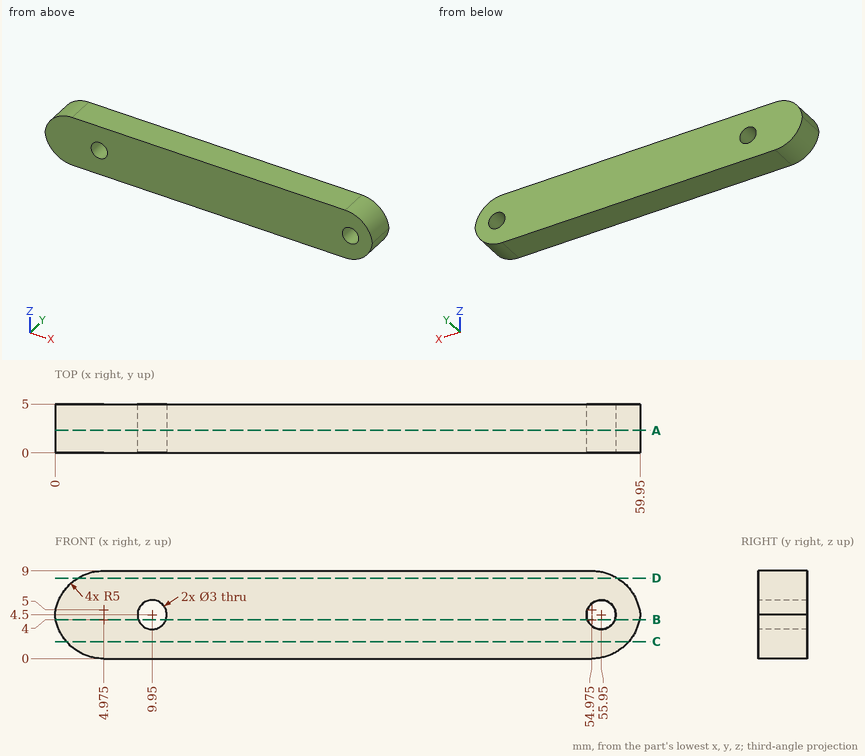
Check sheet for the drawn part. Datum: minimum x, y, z corner. Units: mm. Give positions to 0.01 mm unless a question says otherwise; leave off trailing zeros. Write each loop counter-clockwise with the first axis right and the second up, starting at its lowest first coordinate (ties: lowest second). Pieces come first, ordered by that corner, then holes. Notation, with made-up numbers: M 71,35.5 L 106,35.5 A38 cw 106,74.5 Z; hole C 16.5,-24 d10. An arc over 180 degrees is marked long. One line per question, with ' | ' between items.
1) Gauge pin test, flat ends, axial feed: pin 1 Ø1.5 at (y, z) = (2.5, 7.5) entering from -X; pin 2 Ø5 at (x, z) = (34.5, 5) entering from -Y; pin 3 Ø1.5 at (y, z) = (4.5, 2) entering from -X. Record the tip position at first contact, or that the pin passes through.
Result:
pin 1: stops at x = 0.8 | pin 2: stops at y = 0 | pin 3: stops at x = 0.51
2) Section check C-C on z = 1.75. Enter the section's corners in (x, y), plus the area to 3 significant figures.
Result:
outline: M 1.18,0 L 58.77,0 L 58.77,5 L 1.18,5 Z | area: 288 mm2
3) Section check D-D on z = 8.25. Enter the section's corners in (x, y), plus the area to 3 significant figures.
Result:
outline: M 2.34,0 L 57.61,0 L 57.61,5 L 2.34,5 Z | area: 276 mm2
4) Section check A-A on y = 2.3. Enter the section's corners in (x, z) (3 decimals), plus the area to 3 significant figures.
Result:
outline: M 0,4.5 A5 ccw 4.975,0 L 54.975,0 A5 ccw 59.95,4.5 A5 ccw 54.975,9 L 4.975,9 A5 ccw Z; hole C 9.95,4.5 d3; hole C 55.95,4.5 d3 | area: 504 mm2
5) Section check B-B on z = 4. Enter the section's corners in (x, y).
Result:
outline: M 0.08,0 L 8.54,0 L 8.54,5 L 0.08,5 Z; M 11.36,0 L 54.54,0 L 54.54,5 L 11.36,5 Z; M 57.36,0 L 59.87,0 L 59.87,5 L 57.36,5 Z
6) Thickness scan on line 1 along Z through (x, y) = (10.5, 4.1); line 2 along X through (y, z) = (0.35, 6.25); line 3 along X through (y, z) = (1.3, 8.25). Record the ranges inside material, lowest first. Write a range as [from, to].
Result:
line 1: z = [0, 3.1], [5.9, 9] | line 2: x = [0.51, 59.44] | line 3: x = [2.34, 57.61]
